from build123d import *

# Parameters (mm, degrees)
SKETCH1_R           = 2.35585
BOSS_EXTRUDE1_DEPTH = 7.62


with BuildPart() as part:
    # Sketch1 → Boss-Extrude1 (new body)
    with BuildSketch(Plane(origin=(0, 0, 0), x_dir=(0, 0, -1), z_dir=(1, 0, 0))):
        with BuildLine():
            Line((3.0226, 0), (3.0226, 19.0246))
            Line((3.0226, 19.0246), (2.3876, 19.0246))
            Line((2.3876, 19.0246), (2.3876, 1.853503979))
            ThreePointArc((2.3876, 1.853503979), (-2.137300957, 2.137300957), (-1.853503979, -2.3876))
            Line((-1.853503979, -2.3876), (-20.4724, -2.3876))
            Line((-20.4724, -2.3876), (-20.4724, -3.0226))
            Line((-20.4724, -3.0226), (0, -3.0226))
            ThreePointArc((0, -3.0226), (2.137300957, -2.137300957), (3.0226, 0))
        make_face()
        with Locations(Location((0, 0, 0), (0, 0, 180))):
            Circle(SKETCH1_R, mode=Mode.SUBTRACT)
    extrude(amount=BOSS_EXTRUDE1_DEPTH)


solid = part.part
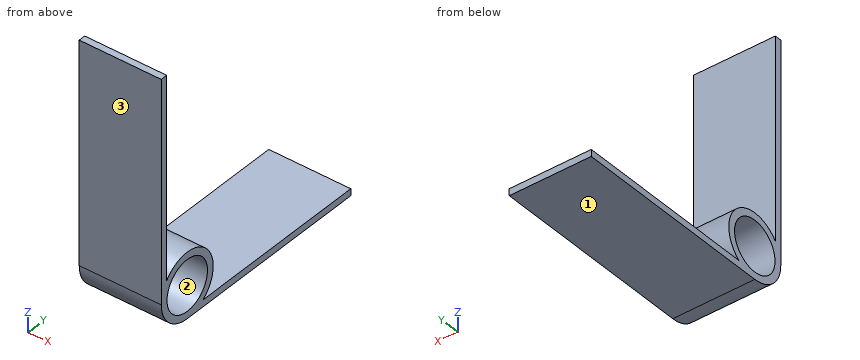
Part model, mm, in its own coordinate system. Face numbers are marked on the shaded views. Give positions to 0.01 mm unless a question says otherwise; leave off trailing zeros. Order: outer loops, then holes, each group sorted by start corner. A loop starts at its lowest first (then second) coordinate and runs counter-clockwise, first axis right, second up. Notation, with made-up numbers: (6.5, 18.25) - (30.5, 18.25) arc R26 ccw to (30.5, 40.25) - close; hole circle Ø9 at (17, 58.5). An arc over 180 degrees is marked (long way). Use a Markdown table: item, result.
1) Saw through at B-B on y = 1. List the corners of the cut face in (x, z).
Checked values:
| item | result |
|---|---|
| outline | (0, -3.02) - (7.62, -3.02) - (7.62, -2.13) - (0, -2.13) - close; (0, 2.13) - (7.62, 2.13) - (7.62, 2.85) - (0, 2.85) - close |
2) Probe L1, parallel to Y at x = 4.25, z = 6; L2, parallel to Z at x = 3, y = -1. List the from-to ranges inside material, lowest first. Write a range as from..to.
Checked values:
| item | result |
|---|---|
| L1 | -3.02..-2.39 |
| L2 | -2.85..-2.13, 2.13..2.85 |
3) Two-plate mould, pull along Z, no slides. Class the marked faces 1, 2 and 3: +Z half, -Z half, draft (parallel to the pull), parting line (faces both ways), or undercut.
Checked values:
| item | result |
|---|---|
| face 1 | -Z half |
| face 2 | undercut |
| face 3 | draft |
4) Saw through at A-A on x = 3.25. List the corners of the cut face in (y, z), plus the area to 3 significant figures.
Checked values:
| item | result |
|---|---|
| outline | (-3.02, 0) arc R3.02 ccw to (0, -3.02) - (19.02, -3.02) - (19.02, -2.39) - (1.85, -2.39) arc R3.02 ccw (long way) to (-2.39, 1.85) - (-2.39, 20.47) - (-3.02, 20.47) - close; hole circle Ø4.71 at (0, 0) |
| area | 34.7 mm² |
5) Flat gauge pins, fed straight in: P1, Ø1.5, axis at x = 1, y = 9, coming from the +Z side; P2, Ø2, axis at x = 3.5, z = 11, coming from the +Y side. Where does each tip first touch, or does it go through?
Checked values:
| item | result |
|---|---|
| P1 | z = -2.39 |
| P2 | y = -2.39 |
6) Saw through at C-C on y = 11.25. List the corners of the cut face in (x, z), plus the area to 3 significant figures.
Checked values:
| item | result |
|---|---|
| outline | (0, -3.02) - (7.62, -3.02) - (7.62, -2.39) - (0, -2.39) - close |
| area | 4.84 mm² |
